Check sheet for the modelled part. Datum: model origin and axes. Units: mm. Coordinates: 2 decimals unless noted, no trailing zeros. Loops run counter-clockwise (first coordinate to the right, second up) from the corner with the lowest first, then second, coordinate; pieces in that order, holes last.
```python
from build123d import *

# Parameters (mm, degrees)
SKETCH1_R                     = 15.875
SKETCH1_R_2                   = 4.7625
BOSS_EXTRUDE1_DEPTH           = 12.7
SKETCH3_W                     = 0.254
SKETCH3_H                     = 0.127
F_001_LINE_CUT_EXTRUDE1_DEPTH = 5.08
F_1_8_0_1250_DOWEL_HOLE1_D    = 3.175


with BuildPart() as part:
    # Sketch1 → Boss-Extrude1 (new body)
    with BuildSketch(Plane.XY):
        Circle(SKETCH1_R)
        Circle(SKETCH1_R_2, mode=Mode.SUBTRACT)
    extrude(amount=-BOSS_EXTRUDE1_DEPTH)

    # Sketch3 → .001 line Cut-Extrude1 (cut)
    with BuildSketch(Plane.XY.offset(-12.7)):
        with Locations((0, 15.8115)):
            Rectangle(SKETCH3_W, SKETCH3_H)
    extrude(amount=F_001_LINE_CUT_EXTRUDE1_DEPTH, mode=Mode.SUBTRACT)

    # 1/8 (0.1250) Dowel Hole1 (through all)
    with Locations(Plane(origin=(0, 0, -12.7), x_dir=(-1, 0, 0), z_dir=(0, 0, -1))):
        with Locations((0, -10.16)):
            Hole(F_1_8_0_1250_DOWEL_HOLE1_D / 2)


solid = part.part
```
1) Mould release check, pull along Y, two halves, no side actions. Record for faces 1 (the cylindrical face through (-3.78, -2.9, -6.26)), 2 (the cylindrical face through (-3.441, -15.497, -6.261)), 3 (the flat face through (3, 4, -12.7)): +Y half, -Y half, draft (parallel to the pull), parting line (faces both ways), or undercut.
Answer sheet:
face 1: undercut
face 2: parting line
face 3: draft
2) Depth check by flat-ended pin: pin 1 (1 mm diameter, centred on x = -5, z = -8, fed in from -Y). Enter the tip coordinate at first touch or a pass-through.
Answer sheet:
pin 1: stops at y = -15.22
3) Section check B-B on x = -3.5. Enter the section's corners in (y, z), plus the area to 3 significant figures.
Answer sheet:
outline: (-15.48, -12.7) - (-3.23, -12.7) - (-3.23, 0) - (-15.48, 0) - close; (3.23, -12.7) - (15.48, -12.7) - (15.48, 0) - (3.23, 0) - close
area: 311 mm2
4) Scan lines: line 1 (Y direction, x = 0, z = -4.75) (1 decimal); line 2 (Y direction, x = 0, z = -8.75) (1 decimal); line 3 (X direction, y = -10.5, z = -9). Record each from-to range of solid material in increasing order.
Answer sheet:
line 1: y = -15.9 to -11.7, -8.6 to -4.8, 4.8 to 15.9
line 2: y = -15.9 to -11.7, -8.6 to -4.8, 4.8 to 15.7
line 3: x = -11.91 to -1.55, 1.55 to 11.91
5) Section check C-C on z = -11.5. Give the number of separate pieces and of enclosed holes in the cut face, plus the area to 3 significant figures.
Answer sheet:
separate pieces: 1
enclosed holes: 2
area: 713 mm2
6) Section check A-A on y = 0. Enter the section's corners in (x, z) (1 decimal), plus the area to 3 significant figures.
Answer sheet:
outline: (-15.9, -12.7) - (-4.8, -12.7) - (-4.8, 0) - (-15.9, 0) - close; (4.8, -12.7) - (15.9, -12.7) - (15.9, 0) - (4.8, 0) - close
area: 282 mm2
